The drawing under review shows one solid part. Ordinate dimensions are in mm from its lowest x, y, z. Coordinates: 2 decimals unless noted, no trailing zeros. Loops run counter-clockwise (first coordinate to the right, second up) from the corner with the lowest first, then second, coordinate; pieces in that order, holes last. Notation, with made-up numbers: (29.25, 51) - (50.25, 51) arc R8 ccw to (50.25, 60) - close; hole circle Ø8 at (-0.75, 19.25). An arc over 180 degrees is marked (long way). Answer as a JSON object with one key per item and string values. Group by question number.
Item 1: We need section B-B (y = 7). Give the boundary of the cut face in (x, z).
Item 2: Clearance check with a flat-ended pin moving along its axis: pin 1 (1.5 mm diameter, centred on x = 3.5, z = 3.5, fed in from -Y). State where the tip first meets the part, or that it passes through.
Item 3: To check wall thickness, follow line 1 (Y direction, x = 7, z = 7.75); line 2 (Y direction, x = 3.5, z = 8.5); line 3 (Z direction, x = 21.5, y = 5). State the ranges of each line that lie inside material, in increasing order.
Item 4: We need section C-C (z = 4.5). Give the boundary of the cut face in (x, y), then the cut area to 3 significant figures.
Item 5: We need section A-A (x = 18.5). Give the boundary of the cut face in (y, z), then the cut area to 3 significant figures.
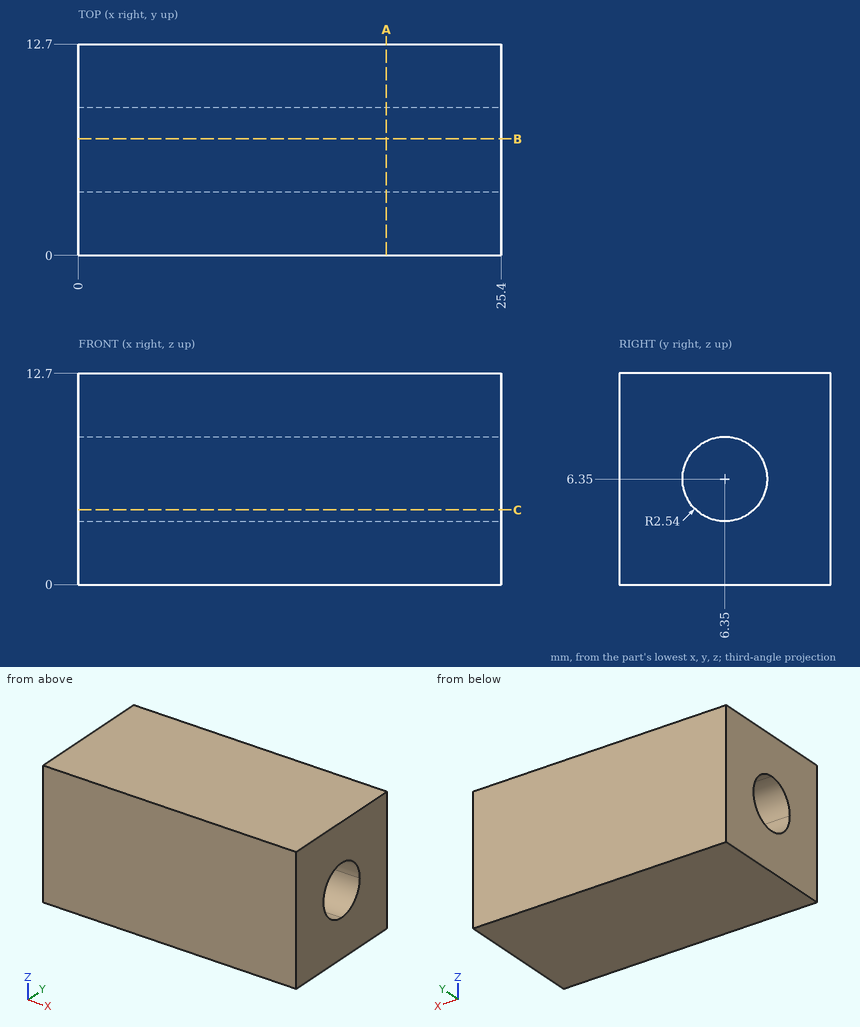
Check sheet entries:
{
 "1": {"outline": "(0, 0) - (25.4, 0) - (25.4, 3.89) - (0, 3.89) - close; (0, 8.81) - (25.4, 8.81) - (25.4, 12.7) - (0, 12.7) - close"},
 "2": {"pin 1": "stops at y = 0"},
 "3": {"line 1": "y = 0 to 4.23, 8.47 to 12.7", "line 2": "y = 0 to 5, 7.7 to 12.7", "line 3": "z = 0 to 4.2, 8.5 to 12.7"},
 "4": {"outline": "(0, 0) - (25.4, 0) - (25.4, 4.61) - (0, 4.61) - close; (0, 8.09) - (25.4, 8.09) - (25.4, 12.7) - (0, 12.7) - close", "area": "234 mm2"},
 "5": {"outline": "(0, 0) - (12.7, 0) - (12.7, 12.7) - (0, 12.7) - close; hole (3.81, 6.35) arc R2.54 ccw to (6.35, 3.81) arc R2.54 ccw to (8.89, 6.35) arc R2.54 ccw to (6.35, 8.89) arc R2.54 ccw to start", "area": "141 mm2"}
}
